Autodesk Inventor part; units mm, degrees
ref_plane "YZ Plane" through (0, 0, 0) normal (1, 0, 0) x (0, 1, 0)
ref_plane "XZ Plane" through (0, 0, 0) normal (0, 1, 0) x (-1, 0, 0)
ref_plane "XY Plane" through (0, 0, 0) normal (0, 0, 1) x (1, 0, 0)
sketch "Sketch1" plane through (0, 0, 0) normal (0, 0, 1) x (1, 0, 0)
  line L0 (25, 0) -> (0, 0)
  line L1 (0, 0) -> (0, 10)
  line L2 (0, 10) -> (5, 10)
  line L3 (25, 0) -> (25, 15)
  circle A0 centre (20, 5) radius 1.6
  line L4 (5, 10) -> (5, 15)
  line L5 (7.5, 15) -> (7.5, 21.731)
  line L6 (7.5, 21.731) -> (5, 21.731)
  line L7 (5, 21.731) -> (5, 26.731)
  line L8 (5, 26.731) -> (20, 26.731)
  line L9 (20, 26.731) -> (20, 21.731)
  line L10 (20, 21.731) -> (15, 21.731)
  line L11 (15, 21.731) -> (15, 15)
  line L12 (5, 15) -> (7.5, 15)
  line L13 (15, 15) -> (25, 15)
  dimension "d0" = 10
  dimension "d8" = 5
  dimension "d9" = 25
  dimension "d12" = 5
  dimension "d13" = 5
  dimension "d20" = 3.2
  dimension "d22" = 7.5
  dimension "d23" = 2.5
  dimension "d24" = 15
  dimension "d25" = 5
  dimension "d26" = 6.731
  dimension "d27" = 15
extrude "Extrusion1" add sketch "Sketch1" along normal blind 6.731
fillet "Fillet1" radius 5 1 edges at (25, 0, 3.3655)
equation "\"d8\" = d3"
equation "\"d12\" = d13"
equation "\"d26\" = THICKB"
equation "\"d15\" = THICKB"
equation "\"THICKA\" = 3.175"
equation "\"THICKB\" = 6.731"
equation "\"THICKC\" = 12.7"
equation "\"MAGDIA\" = 9.5"
equation "\"BALLDIA\" = 12"
properties part number "Carriage_Belt_Lock"
Build history of the part. All positions in model axes, mm. A direction names the side the tool comes from. Give positions to 0.01 mm unless a question says otherwise; leave off trailing zeros. Loops run counter-clockwise (first coordinate to the right, second up) from the corner with the lowest first, then second, coordinate; pieces in that order, holes last.
Item 1: Slice it at A-A, the plane x = 15.5. List the corners of the cut face in (y, z), and give its area (3 significant figures).
Answers follow:
outline: (0, 0) - (15, 0) - (15, 6.73) - (0, 6.73) - close; (21.73, 0) - (26.73, 0) - (26.73, 6.73) - (21.73, 6.73) - close
area: 135 mm2
Item 2: Drill centre lines: line 1 (X direction, y = 25.5, z = 3); line 2 (X direction, y = 12.25, z = 6.25); line 3 (Y direction, x = 2, z = 3). Where is each one in solid material? Low to high.
Answers follow:
line 1: x = 5 to 20
line 2: x = 5 to 25
line 3: y = 0 to 10
Item 3: Which spindle directions (+Z, -Z, +X, -X, +Y, -Y) get a long thin tool onto all of the face, cutting with end or side? Do faces 1 (the face through (5, 24, 3)), 2 (the face through (20, 24, 3)), 3 (the face through (18, 21.731, 3)), 4 (the face through (6, 15, 3)). Say none if no direction does.
Answers follow:
face 1: +Z, -Z, -X, +Y
face 2: +Z, -Z, +X, +Y
face 3: +Z, -Z, +X
face 4: +Z, -Z, -X
Item 4: Slice it at D-D, the plane x = 4.5. List the corners of the cut face in (y, z).
Answers follow:
outline: (0, 0) - (10, 0) - (10, 6.73) - (0, 6.73) - close
Item 5: Flat gauge pins, fed straight in: pin 1 (1.5 mm diameter, centred on y = 13, z = 4.5, fed in from -X); pin 2 (2 mm diameter, centred on y = 17.5, z = 3, fed in from +X); pin 3 (4 mm diameter, centred on y = 25, z = 2.5, fed in from +X); pin 4 (1.9 mm diameter, centred on x = 20, y = 5, fed in from +Z). Where does each tip first touch, or does it go through?
Answers follow:
pin 1: stops at x = 5
pin 2: stops at x = 15
pin 3: stops at x = 20
pin 4: passes through
Item 6: Slice it at C-C, the plane y = 6.25. List the corners of the cut face in (x, z).
Answers follow:
outline: (0, 0) - (19, 0) - (19, 6.73) - (0, 6.73) - close; (21, 0) - (25, 0) - (25, 6.73) - (21, 6.73) - close
Item 7: Pull direction X, two halves, no side cores. Call faces 5 (the face through (2, 10, 3)), 6 (the face through (18.82, 3.92, 3.32)), 7 (the face through (0, 5, 3)): released by +X, released by -X, zero draft, split by the parting line, or undercut.
Answers follow:
face 5: zero draft
face 6: undercut
face 7: released by -X
Item 8: Slice it at B-B, the plane z = 4.5. List the corners of the cut face in (x, y), and give its area (3 significant figures).
Answers follow:
outline: (0, 0) - (20, 0) arc R5 ccw to (25, 5) - (25, 15) - (15, 15) - (15, 21.73) - (20, 21.73) - (20, 26.73) - (5, 26.73) - (5, 21.73) - (7.5, 21.73) - (7.5, 15) - (5, 15) - (5, 10) - (0, 10) - close; hole circle Ø3.2 at (20, 5)
area: 462 mm2
